from build123d import *

# Parameters (mm, degrees)
REVOLVE1_ANGLE      = 180
SKETCH3_R           = 25.457715114
BOSS_EXTRUDE1_DEPTH = 5
SKETCH4_R           = 22
BOSS_EXTRUDE2_DEPTH = 12
SKETCH5_R           = 25
BOSS_EXTRUDE3_DEPTH = 3.5
SKETCH6_R           = 19.5
CUT_EXTRUDE1_DEPTH  = 17


with BuildPart() as part:
    # Sketch1 → Revolve1 (revolve)
    with BuildSketch(Plane(origin=(0, 0, 0), x_dir=(1, 0, 0), z_dir=(0, 1, 0))):
        with BuildLine():
            Line((-0.996315138, 27.481946004), (0.996315138, -27.481946004))
            ThreePointArc((0.996315138, -27.481946004), (27.481946004, 0.996315138), (-0.996315138, 27.481946004))
        make_face()
    revolve(axis=Axis((-0.996315138, 0, -27.481946004), (0.036229641, 0, 0.999343491)), revolution_arc=REVOLVE1_ANGLE)

    # Sketch2 → Cut-Revolve1 (revolve, cut)
    with BuildSketch(Plane.XZ):
        with BuildLine():
            Line((0, 25), (0, -25))
            ThreePointArc((0, -25), (25, 0), (0, 25))
        make_face()
    revolve(axis=Axis((0, 0, 25), (0, 0, -1)), mode=Mode.SUBTRACT)

    # Sketch3 → Boss-Extrude1 (add)
    with BuildSketch(Plane.XZ):
        Circle(SKETCH3_R)
    extrude(amount=-BOSS_EXTRUDE1_DEPTH)

    # Sketch4 → Boss-Extrude2 (add)
    with BuildSketch(Plane.XZ):
        Circle(SKETCH4_R)
    extrude(amount=BOSS_EXTRUDE2_DEPTH)

    # Sketch5 → Boss-Extrude3 (add)
    with BuildSketch(Plane.XZ.offset(12)):
        Circle(SKETCH5_R)
    extrude(amount=-BOSS_EXTRUDE3_DEPTH)

    # Sketch6 → Cut-Extrude1 (cut)
    with BuildSketch(Plane.XZ.offset(12)):
        Circle(SKETCH6_R)
    extrude(amount=-CUT_EXTRUDE1_DEPTH, mode=Mode.SUBTRACT)


solid = part.part
Model file for the job. Use its own axes, mm. A direction names the side the tool comes from. Give positions to 0.01 mm unless a question says otherwise; leave off trailing zeros. Write each loop counter-clockwise with the first axis right and the second up, starting at its lowest first coordinate (ties: lowest second). Pieces come first, ordered by that corner, then holes. Notation, with made-up numbers: M 26.25,-36 L 65.25,-36 A9 ccw 65.25,-21 Z; hole C 60.5,-18 d8. An arc over 180 degrees is marked long. One line per item, written item: value. Start each with the question number.
Q1. Drop flat-ended pins along their axis: pin 1 Ø5 at (x, z) = (-16.5, 22) entering from +Y; pin 2 Ø4 at (x, z) = (22, -15.5) entering from +Y; pin 3 Ø1 at (x, y) = (-14, 12) entering from -Z. Give the stop position or say it passes through.
Q2. 3-axis set-ups, long thin cutter, end or side, ignore diameter. For faces 1 (the flat face through (-16.44, 5, -10.77)), 2 (the cylindrical face through (23.846, -10.274, 7.509)), 3 (the flat face through (15, -12, -13)): which of +Z, -Z, +X, -X, +Y, -Y reach the whole face in a straight line?
Q3. Saw through at B-B, the plane z = 0. Write the cut outline in (x, y), plus the area to 3 significant figures.
Q4. Saw through at C-C, the plane y = -4.5. Write the cut outline in (x, z).
Q5. Saw through at A-A, the plane x = 0. Write the cut outline in (y, z).
Q6. Saw through at D-D, the plane y = 19.5. Write the cut outline in (x, z), plus the area to 3 significant figures.
Q7. Probe probe 1 along Z at (x, y) = (0, -6.25); probe 2 along Y at (x, z) = (10.5, 20); probe 3 along Y at (x, z) = (-21.5, 8). List the from-to ranges inside material, lowest first. Write a range as [from, to].
Q8. Two-plate mould, pull along Z, no slides. Class faces 4 (the flat face through (-12.4, 0, -18.5)), 5 (the cylindrical face through (-4.769, -4.19, -21.477)), 6 (the cylindrical face through (-2.539, -3.619, 19.334)): +Z half, -Z half, draft (parallel to the pull), parting line (faces both ways), or undercut.
Output values:
1. pin 1: stops at y = 11.46
1. pin 2: stops at y = 11.65
1. pin 3: stops at z = -20.84
2. face 1: none
2. face 2: -Y
2. face 3: +Z, -Z, +X, -X, -Y
3. outline: M -27.5,0 L -22,0 L -22,-8.5 L -25,-8.5 L -25,-12 L -19.5,-12 L -19.5,5 L -24.49,5 A25 cw 24.49,5 L 19.5,5 L 19.5,-12 L 25,-12 L 25,-8.5 L 22,-8.5 L 22,0 L 27.5,0 A27.5 ccw Z
3. area: 340 mm²
4. outline: C 0,0 d44; hole C 0,0 d39
5. outline: M -12,-25 L -8.5,-25 L -8.5,-22 L 0,-22 L 0,-27.5 A27.5 ccw 0,27.5 L 0,22 L -8.5,22 L -8.5,25 L -12,25 L -12,19.5 L 5,19.5 L 5,24.49 A25 cw 5,-24.49 L 5,-19.5 L -12,-19.5 Z
6. outline: C 0,0 d38.78; hole C 0,0 d31.29
6. area: 412 mm²
7. probe 1: z = [-22, -19.5], [19.5, 22]
7. probe 2: y = [-12, -8.5], [0, 5], [10.71, 15.68]
7. probe 3: y = [-12, -8.5], [0, 5], [9.94, 15.17]
8. face 4: draft
8. face 5: parting line
8. face 6: undercut
